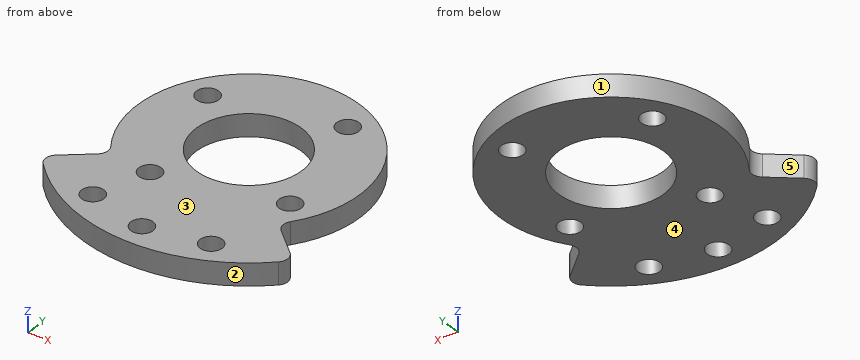
from build123d import *

# Parameters (mm, degrees)
SKETCH_1_R           = 20
SKETCH_1_R_2         = 2
EXTRUDE_1_DEPTH      = 4
EXTRUDE_START        = -4
EXTRUDE_2_DEPTH      = 4
FILLET_2_R           = 5
FILLET_3_R           = 5
SKETCH_3_R           = 58.160089131
SKETCH_3_R_2         = 39.60449563
CUT_EXTRUDE_1_DEPTH  = 4
FILLET_4_R           = 8
EXTRUDE_3_DEPTH      = 4
SKETCH_5_R           = 2
CUT_EXTRUDE_2_DEPTH  = 4
SKETCH_6_R           = 2
CUT_EXTRUDE_3_DEPTH  = 10
EXTRUDE_4_DEPTH      = 4
EXTRUDE_6_DEPTH      = 4
CUT_EXTRUDE_6_DEPTH  = 4
FILLET_6_R           = 10
FILLET_7_R           = 10
FILLET_8_R           = 10
SKETCH_10_R          = 2
EXTRUDE_7_DEPTH      = 4
SKETCH_11_R          = 55.332509923
SKETCH_11_R_2        = 30
CUT_EXTRUDE_7_DEPTH  = 4
EXTRUDE_8_DEPTH      = 4
SKETCH_13_R          = 2
CUT_EXTRUDE_8_DEPTH  = 4
SKETCH_14_R          = 9.5
CUT_EXTRUDE_9_DEPTH  = 10
SKETCH_15_R          = 2
EXTRUDE_9_DEPTH      = 5
SKETCH_16_R          = 20
SKETCH_16_R_2        = 9.5
EXTRUDE_10_DEPTH     = 4
SKETCH_18_R          = 2
CUT_EXTRUDE_11_DEPTH = 39.776527497
FILLET_9_R           = 2
FILLET_10_R          = 2
CUT_EXTRUDE_START    = -5
SKETCH_19_R          = 2
CUT_EXTRUDE_12_DEPTH = 5


with BuildPart() as part:
    # 草图1 → 凸台-拉伸1 (new body)
    with BuildSketch(Plane.XY):
        Circle(SKETCH_1_R)
        with Locations((-15.5, 0)):
            Circle(SKETCH_1_R_2, mode=Mode.SUBTRACT)
        with Locations((15.5, 0)):
            Circle(SKETCH_1_R_2, mode=Mode.SUBTRACT)
        with Locations((-7.75, 13.423393759)):
            Circle(SKETCH_1_R_2, mode=Mode.SUBTRACT)
        with Locations((-7.75, -13.423393759)):
            Circle(SKETCH_1_R_2, mode=Mode.SUBTRACT)
        with Locations((7.75, -13.423393759)):
            Circle(SKETCH_1_R_2, mode=Mode.SUBTRACT)
        with Locations((7.75, 13.423393759)):
            Circle(SKETCH_1_R_2, mode=Mode.SUBTRACT)
    extrude(amount=EXTRUDE_1_DEPTH)

    # 草图2 → 凸台-拉伸2 (add)
    with BuildSketch(Plane.XY.offset(4).offset(EXTRUDE_START)):
        with BuildLine():
            add(Edge.make_bspline(
                [(-31.652235688, -31.652235688), (-33.388516019, -22.659494294), (-23.392443281, -20.962737075), (-16.1166561, -16.161254448), (-15.240575556, -12.950863166)],
                knots=[0, 0, 0, 0, 0.575012139, 0.86884139, 0.86884139, 0.86884139, 0.86884139], degree=3))
            ThreePointArc((-31.652235688, -31.652235688), (0, -44.76302099), (31.652235688, -31.652235688))
            add(Edge.make_bspline(
                [(31.652235688, -31.652235688), (33.388516019, -22.659494294), (23.392443281, -20.962737075), (16.1166561, -16.161254448), (15.240575556, -12.950863166)],
                knots=[0, 0, 0, 0, 0.575012139, 0.86884139, 0.86884139, 0.86884139, 0.86884139], degree=3))
            ThreePointArc((15.240575556, -12.950863166), (0, -20), (-15.240575556, -12.950863166))
        make_face()
    extrude(amount=EXTRUDE_2_DEPTH)

    # 圆角2
    fillet_2_edges = [part.edges().sort_by_distance(p)[0] for p in [
        (-31.652235688, -31.652235688, 2),
    ]]
    fillet(fillet_2_edges, radius=FILLET_2_R)

    # 圆角3
    fillet_3_edges = [part.edges().sort_by_distance(p)[0] for p in [
        (31.652235688, -31.652235688, 2),
    ]]
    fillet(fillet_3_edges, radius=FILLET_3_R)

    # 草图3 → 切除-拉伸1 (cut)
    with BuildSketch(Plane(origin=(0, 0, 0), x_dir=(-1, 0, 0), z_dir=(0, 0, -1))):
        Circle(SKETCH_3_R)
        Circle(SKETCH_3_R_2, mode=Mode.SUBTRACT)
    extrude(amount=-CUT_EXTRUDE_1_DEPTH, mode=Mode.SUBTRACT)

    # 圆角4
    fillet_4_edges = [part.edges().sort_by_distance(p)[0] for p in [
        (30.87581987, -24.803221997, 2),
        (-30.87581987, -24.803221997, 2),
    ]]
    fillet(fillet_4_edges, radius=FILLET_4_R)

    # 草图4 → 凸台-拉伸3 (add)
    with BuildSketch(Plane(origin=(0, 0, 0), x_dir=(-1, 0, 0), z_dir=(0, 0, -1))):
        with BuildLine():
            Line((-22.183787779, -32.808468935), (-22.405322857, -33.136105801))
            ThreePointArc((-22.405322857, -33.136105801), (0.038199329, -39.99998176), (22.468570811, -33.093251967))
            Line((22.468570811, -33.093251967), (22.183787779, -32.808468935))
            ThreePointArc((22.183787779, -32.808468935), (0, -39.60449563), (-22.183787779, -32.808468935))
        make_face()
    extrude(amount=-EXTRUDE_3_DEPTH)

    # 草图5 → 切除-拉伸2 (cut)
    with BuildSketch(Plane(origin=(0, 0, 0), x_dir=(-1, 0, 0), z_dir=(0, 0, -1))):
        with Locations((-15.848184815, -33.986542014)):
            Circle(SKETCH_5_R)
        with Locations((0, -37.5)):
            Circle(SKETCH_5_R)
        with Locations(Location((15.848184815, -33.986542014, 0), (0, 0, 180))):
            Circle(SKETCH_5_R)
    extrude(amount=-CUT_EXTRUDE_2_DEPTH, mode=Mode.SUBTRACT)

    # 草图6 → 切除-拉伸3 (cut)
    with BuildSketch(Plane(origin=(0, 0, 0), x_dir=(-1, 0, 0), z_dir=(0, 0, -1))):
        with Locations((0.038199329, -29.99998176)):
            Circle(SKETCH_6_R)
    extrude(amount=-CUT_EXTRUDE_3_DEPTH, mode=Mode.SUBTRACT)

    # 草图7 → 凸台-拉伸4 (add)
    with BuildSketch(Plane.XY.offset(4)):
        with BuildLine():
            Line((-22.468570811, -33.093251967), (-23.907156981, -34.531838137))
            ThreePointArc((-23.907156981, -34.531838137), (-0.231167262, -41.999363825), (23.525589, -34.792911091))
            Line((23.525589, -34.792911091), (22.405322857, -33.136105801))
            Line((22.405322857, -33.136105801), (22.183787779, -32.808468935))
            ThreePointArc((22.183787779, -32.808468935), (0, -39.60449563), (-22.183787779, -32.808468935))
            Line((-22.183787779, -32.808468935), (-22.468570811, -33.093251967))
        make_face()
    extrude(amount=-EXTRUDE_4_DEPTH)

    # 草图8 → 凸台-拉伸6 (add)
    with BuildSketch(Plane(origin=(0, 0, 0), x_dir=(-1, 0, 0), z_dir=(0, 0, -1))):
        with BuildLine():
            Line((-25.678439695, -25.558394246), (-20.516854663, -32.863070329))
            Line((-20.516854663, -32.863070329), (-23.525589, -34.792911091))
            add(Edge.make_bspline(
                [(-23.525589, -34.792911091), (-26.001835591, -30.056258517), (-25.678439695, -25.558394246)],
                knots=[0, 0, 0, 0.47951431, 0.47951431, 0.47951431], degree=2))
        make_face()
        with BuildLine():
            Line((20.516854663, -32.863070329), (23.525589, -34.792911091))
            add(Edge.make_bspline(
                [(23.525589, -34.792911091), (26.001835591, -30.056258517), (25.678439695, -25.558394246)],
                knots=[0, 0, 0, 0.47951431, 0.47951431, 0.47951431], degree=2))
            Line((25.678439695, -25.558394246), (20.516854663, -32.863070329))
        make_face()
    extrude(amount=-EXTRUDE_6_DEPTH)

    # 草图9 → 切除-拉伸6 (cut)
    with BuildSketch(Plane(origin=(0, 0, 0), x_dir=(-1, 0, 0), z_dir=(0, 0, -1))):
        Polygon((23.742659966, -34.367341122), (22.906265437, -35.20373565), (24.433492861, -34.374984505), align=None)
    extrude(amount=-CUT_EXTRUDE_6_DEPTH, mode=Mode.SUBTRACT)

    # 圆角6
    fillet_6_edges = [part.edges().sort_by_distance(p)[0] for p in [
        (23.525589, -34.792911091, 2),
    ]]
    fillet(fillet_6_edges, radius=FILLET_6_R)

    # 圆角7
    # the kernel refuses this fillet: 10 mm, written as the material it takes off along each edge
    with BuildSketch(Plane(origin=(-23.742659966, -34.367341122, 10.292446297), x_dir=(0.7071067812003878, -0.7071067811727072, 0), z_dir=(0, 0, -1))) as fillet_7_piece_1:
        with BuildLine():
            CenterArc((1.956172782, -9.970053017), FILLET_7_R, 94.435296014, 20.980736708)
            Line((-2.335706132, -0.937900705), (-2.42154371, -0.757257658))
            ThreePointArc((-2.42154371, -0.757257658), (-1.256201499, -0.248323162), (-0.06365122, 0.189600955))
            Line((-0.06365122, 0.189600955), (0, 0.2))
            ThreePointArc((0, 0.2), (0.591420243, 0.2), (1.16737384, 0.19940106))
            Line((1.16737384, 0.19940106), (1.182840486, 0))
        make_face()
    extrude(amount=16.584892581, mode=Mode.SUBTRACT)

    # 圆角8
    fillet_8_edges = [part.edges().sort_by_distance(p)[0] for p in [
        (-22.906265437, -35.20373565, 2),
    ]]
    fillet(fillet_8_edges, radius=FILLET_8_R)

    # 草图10 → 凸台-拉伸7 (add)
    with BuildSketch(Plane(origin=(0, 0, 0), x_dir=(-1, 0, 0), z_dir=(0, 0, -1))):
        with Locations((0.038199329, -29.99998176)):
            Circle(SKETCH_10_R)
        with Locations((0, -37.5)):
            Circle(SKETCH_10_R)
        with Locations((15.848184815, -33.986542014)):
            Circle(SKETCH_10_R)
        with Locations((-15.848184815, -33.986542014)):
            Circle(SKETCH_10_R)
    extrude(amount=-EXTRUDE_7_DEPTH)

    # 草图11 → 切除-拉伸7 (cut)
    with BuildSketch(Plane(origin=(0, 0, 0), x_dir=(-1, 0, 0), z_dir=(0, 0, -1))):
        Circle(SKETCH_11_R)
        Circle(SKETCH_11_R_2, mode=Mode.SUBTRACT)
    extrude(amount=-CUT_EXTRUDE_7_DEPTH, mode=Mode.SUBTRACT)

    # 草图12 → 凸台-拉伸8 (add)
    with BuildSketch(Plane(origin=(0, 0, 0), x_dir=(-1, 0, 0), z_dir=(0, 0, -1))):
        with BuildLine():
            Line((-15.240575556, -12.950863166), (-22.860863333, -19.426294749))
            ThreePointArc((-22.860863333, -19.426294749), (-19.109156974, -23.126610641), (-14.767877105, -26.1134028))
            Line((-14.767877105, -26.1134028), (-15.240575556, -12.950863166))
        make_face()
        with BuildLine():
            Line((15.240575556, -12.950863166), (14.767877105, -26.1134028))
            ThreePointArc((14.767877105, -26.1134028), (19.109156974, -23.126610641), (22.860863333, -19.426294749))
            Line((22.860863333, -19.426294749), (15.240575556, -12.950863166))
        make_face()
    extrude(amount=-EXTRUDE_8_DEPTH)

    # 草图13 → 切除-拉伸8 (cut)
    with BuildSketch(Plane(origin=(0, 0, 0), x_dir=(-1, 0, 0), z_dir=(0, 0, -1))):
        with Locations((-10.776765674, -23.110848569)):
            Circle(SKETCH_13_R)
        with Locations((0, -25.5)):
            Circle(SKETCH_13_R)
        with Locations(Location((10.776765674, -23.110848569, 0), (0, 0, 180))):
            Circle(SKETCH_13_R)
    extrude(amount=-CUT_EXTRUDE_8_DEPTH, mode=Mode.SUBTRACT)

    # 草图14 → 切除-拉伸9 (cut)
    with BuildSketch(Plane(origin=(0, 0, 0), x_dir=(-1, 0, 0), z_dir=(0, 0, -1))):
        Circle(SKETCH_14_R)
    extrude(amount=-CUT_EXTRUDE_9_DEPTH, mode=Mode.SUBTRACT)

    # 草图15 → 凸台-拉伸9 (add)
    with BuildSketch(Plane(origin=(0, 0, 0), x_dir=(-1, 0, 0), z_dir=(0, 0, -1))):
        with Locations(Location((0, 15.5, 0), (0, 0, 180))):
            Circle(SKETCH_15_R)
        with Locations(Location((0, -15.5, 0), (0, 0, 180))):
            Circle(SKETCH_15_R)
        with Locations(Location((-13.423393758, 7.75, 0), (0, 0, 180))):
            Circle(SKETCH_15_R)
        with Locations(Location((13.423393759, 7.75, 0), (0, 0, 180))):
            Circle(SKETCH_15_R)
        with Locations(Location((13.423393759, -7.75, 0), (0, 0, 180))):
            Circle(SKETCH_15_R)
        with Locations(Location((-13.423393758, -7.75, 0), (0, 0, 180))):
            Circle(SKETCH_15_R)
    extrude(amount=EXTRUDE_9_DEPTH)

    # 草图16 → 凸台-拉伸10 (add)
    with BuildSketch(Plane.XY.offset(4).offset(EXTRUDE_START)):
        Circle(SKETCH_16_R)
        with Locations(Location((0, 0, 0), (0, 0, 180))):
            Circle(SKETCH_16_R_2, mode=Mode.SUBTRACT)
    extrude(amount=EXTRUDE_10_DEPTH)

    # 草图18 → 切除-拉伸11 (cut, through all)
    with BuildSketch(Plane(origin=(0, 0, -5), x_dir=(-1, 0, 0), z_dir=(0, 0, -1))):
        with Locations((13.423393759, 7.75)):
            Circle(SKETCH_18_R)
        with Locations((7.75, -13.423393759)):
            Circle(SKETCH_18_R)
        with Locations((-13.423393759, -7.75)):
            Circle(SKETCH_18_R)
        with Locations((-7.75, 13.423393759)):
            Circle(SKETCH_18_R)
    extrude(amount=-CUT_EXTRUDE_11_DEPTH, mode=Mode.SUBTRACT)

    # 圆角9
    fillet_9_edges = [part.edges().sort_by_distance(p)[0] for p in [
        (-15.240575556, -12.950863166, 2),
        (15.240575556, -12.950863166, 2),
    ]]
    fillet(fillet_9_edges, radius=FILLET_9_R)

    # 圆角10
    fillet_10_edges = [part.edges().sort_by_distance(p)[0] for p in [
        (22.860863333, -19.426294749, 2),
        (-22.860863333, -19.426294749, 2),
    ]]
    fillet(fillet_10_edges, radius=FILLET_10_R)

    # 草图19 → 切除-拉伸12 (cut)
    with BuildSketch(Plane(origin=(0, 0, -5), x_dir=(-1, 0, 0), z_dir=(0, 0, -1)).offset(CUT_EXTRUDE_START)):
        with Locations((0, 15.5)):
            Circle(SKETCH_19_R)
        with Locations((0, -15.5)):
            Circle(SKETCH_19_R)
        with Locations((13.423393759, -7.75)):
            Circle(SKETCH_19_R)
        with Locations((-13.423393758, 7.75)):
            Circle(SKETCH_19_R)
    extrude(amount=CUT_EXTRUDE_12_DEPTH, mode=Mode.SUBTRACT)


solid = part.part
Source: CAD feature listing. Evaluate the final solid. Frame: model axes, mm. Face numbers are marked on the shaded views. A direction names the side the tool comes from. Give positions to 0.01 mm unless a question says otherwise; leave off trailing zeros. Order: outer loops, then holes, each group sorted by start corner. A loop starts at its lowest first (then second) coordinate and runs counter-clockwise, first axis right, second up. Notation, with made-up numbers: (3.5, 41) -> (50.5, 41) arc R34 cw to (50.5, 73) -> close; hole circle Ø10 at (32.25, 24.25). An arc over 180 degrees is marked (long way). Use a Markdown table: item, result.
1) Section query D-D, the plane z = 1.9. Count the separate pieces of the cut face and the enclosed holes in it, then the cut area to 3 significant figures.
Answer list:
| item | result |
|---|---|
| separate pieces | 1 |
| enclosed holes | 8 |
| area | 1,320 mm² |
2) Ray query, line 1 along Y through (x, z) = (0, 1.5); line 2 along Y through (x, z) = (6, 0.5); line 3 along Y through (x, z) = (-5, 1.6). Return the intervals inside material, ascending. Write a range as [from, to].
Answer list:
| item | result |
|---|---|
| line 1 | [-30, -27.5], [-23.5, -9.5], [9.5, 20] |
| line 2 | [-29.39, -7.37], [7.37, 12.46], [14.39, 19.08] |
| line 3 | [-29.58, -8.08], [8.08, 19.36] |
3) Section query A-A, the plane x = 0. Return the cut outline in (y, z).
Answer list:
| item | result |
|---|---|
| outline | (-30, 0) -> (-27.5, 0) -> (-27.5, 4) -> (-30, 4) -> close; (-23.5, 0) -> (-9.5, 0) -> (-9.5, 4) -> (-23.5, 4) -> close; (9.5, 0) -> (20, 0) -> (20, 4) -> (9.5, 4) -> close |
4) Section query B-B, the plane y = 0. Return the cut outline in (x, z).
Answer list:
| item | result |
|---|---|
| outline | (-20, 0) -> (-9.5, 0) -> (-9.5, 4) -> (-20, 4) -> close; (9.5, 0) -> (20, 0) -> (20, 4) -> (9.5, 4) -> close |
5) Mould query, pull axis Y, two halves, no side actions, for the marked faces 1, 2 and 3. Classes: +Y half, -Y half, draft (parallel to the pull), parting line (faces both ways), or undercut.
Answer list:
| item | result |
|---|---|
| face 1 | undercut |
| face 2 | -Y half |
| face 3 | draft |
6) Reachability of the marked faces 4 and 5 from +Z, -Z, +X, -X, +Y, -Y: full face, straight path, thin tool, end or side. Return the list, or none.
Answer list:
| item | result |
|---|---|
| face 4 | -Z, +X, -X, +Y, -Y |
| face 5 | +Z, -Z, -X |
7) Contact query for flat-ended pins moving along their axis: P1, Ø4.5, axis at x = 10.78, y = -23.11, coming from the +Z side; P2, Ø1.5, axis at y = 5, z = 1, coming from the +X side; P3, Ø1.5, axis at y = 5.5, z = 3, coming from the -X side. Output: stop coordinate, or through.
Answer list:
| item | result |
|---|---|
| P1 | z = 4 |
| P2 | x = 19.54 |
| P3 | x = -19.43 |
8) Section query C-C, the plane y = -22.5. Return the cut outline in (x, z), then the cut area to 3 significant figures.
Answer list:
| item | result |
|---|---|
| outline | (-19.84, 0) -> (-12.68, 0) -> (-12.68, 4) -> (-19.84, 4) -> close; (-8.87, 0) -> (8.87, 0) -> (8.87, 4) -> (-8.87, 4) -> close; (12.68, 0) -> (19.84, 0) -> (19.84, 4) -> (12.68, 4) -> close |
| area | 128 mm² |
